```python
from build123d import *

# Parameters (mm, degrees)
F1_DEPTH = 6.35
F4_DEPTH = 6.35


with BuildPart() as f1:
    # F0 (on Top) → F1 (new body)
    with BuildSketch(Plane.XY):
        Polygon((12.7, -7.3323484187), (12.7, 7.3323484187), (0, 14.6646968374), (-12.7, 7.3323484187), (-12.7, -7.3323484187), (0, -14.6646968374), align=None)
    extrude(amount=F1_DEPTH)

    # F3 (on face) → F4 (join, through all)
    with BuildSketch(Plane(origin=(0, 0, 0), x_dir=(1, 0, 0), z_dir=(0, 0, -1))):
        with BuildLine():
            ThreePointArc((4.3930360984, 12.1283762634), (6.2703188288, 14.5276326774), (6.9390436724, 17.4997411668))
            ThreePointArc((6.9390436724, 17.4997411668), (-2.9721084894, 23.7700599956), (-4.3930360984, 12.1283762634))
            Line((-4.3930360984, 12.1283762634), (-1.9827005664, 13.5199841317))
            ThreePointArc((-1.9827005664, 13.5199841317), (-2.3402873387, 21.2802996927), (4.4462981901, 17.4997411668))
            ThreePointArc((4.4462981901, 17.4997411668), (3.7805585258, 15.1594538282), (1.9827005664, 13.5199841317))
            Line((1.9827005664, 13.5199841317), (4.3930360984, 12.1283762634))
        make_face()
    extrude(amount=-F4_DEPTH)


solid = f1.part
```
Source: CAD feature listing. Evaluate the final solid. Frame: model axes, mm. A direction names the side the tool comes from. Round coordinates to 2 decimals unless told otherwise and drop trailing zeros. Write each loop counter-clockwise with the first axis right and the second up, starting at its lowest first coordinate (ties: lowest second). Pieces come first, ordered by that corner, then holes. Notation, with made-up numbers: M -20,31.5 L -16,31.5 A31 cw -16,60.5 Z; hole C 23,53.25 d6. An arc over 180 degrees is marked long. Answer as a JSON object with one key per item and string values. Group by question number.
(1) Section query A-A on z = 5.5. Output: boundary loops of the cut face in (x, y), then the cut area to 3 significant figures.
(2) Section query D-D on x = 8.75. Output: boundary loops of the cut face in (y, z), then the cut area to 3 significant figures.
(3) Mould query, pull axis X, two halves, no side actions, for faces 4 (the flat face through (0.98, -14.1, 3.13)), 5 (the flat face through (0, 0, 0)), 6 (the flat face through (-1.01, -14.08, 3.13)), 7 (the flat face through (12.7, 0, 3)). Classes: +X half, -X half, draft (parallel to the pull), parting line (faces both ways), or undercut.
(4) First-contact query: pin 1 (1.5 mm diameter, centred on x = 3.5, z = 3.5, fed in from -Y); pin 2 (1 mm diameter, centred on x = 1.5, z = 0.5, fed in from +Y). Flat tips, straight axial feed; report the tip coordinate or a pass-through.
(5) Section query B-B on x = 0.5. Output: boundary loops of the cut face in (y, z).
(6) Section query C-C on x = -9.25. Output: boundary loops of the cut face in (y, z), then the cut area to 3 significant figures.
(7) Ray query, line 1 (Y direction, x = 0, z = 2.75); line 2 (X direction, y = -20, z = 4); line 3 (Y direction, x = 2.25, z = 1.25). Return the intervals inside material, ascending. Write a range as [from, to].
(8) Reachability of faces 1 (the flat face through (-8.6, -9.7, 3.1)), 2 (the flat face through (-6.26, 11.05, 3.13)), 3 (the flat face through (8.488, -9.764, 3.131)) from +Z, -Z, +X, -X, +Y, -Y: full face, straight path, thin tool, end or side. Return the list, or none.
Computed values:
{
 "1": {"outline": "M -12.7,-7.33 L -4.39,-12.13 A6.94 ccw long 4.39,-12.13 L 12.7,-7.33 L 12.7,7.33 L 0,14.66 L -12.7,7.33 Z; hole M -1.98,-13.52 A4.45 ccw long 1.98,-13.52 L 0,-14.66 Z", "area": "631 mm^2"},
 "2": {"outline": "M -9.61,0 L 9.61,0 L 9.61,6.35 L -9.61,6.35 Z", "area": "122 mm^2"},
 "3": {"face 4": "undercut", "face 5": "draft", "face 6": "undercut", "face 7": "+X half"},
 "4": {"pin 1": "y = -23.87", "pin 2": "y = 14.09"},
 "5": {"outline": "M -24.42,0 L -21.92,0 L -21.92,6.35 L -24.42,6.35 Z; M -14.38,0 L 14.38,0 L 14.38,6.35 L -14.38,6.35 Z"},
 "6": {"outline": "M -9.32,0 L 9.32,0 L 9.32,6.35 L -9.32,6.35 Z", "area": "118 mm^2"},
 "7": {"line 1": "[-24.44, -21.95], [-14.66, 14.66]", "line 2": "[-6.47, -3.68], [3.68, 6.47]", "line 3": "[-24.06, -21.33], [-13.66, 13.37]"},
 "8": {"face 1": "+Z, -Z, -X", "face 2": "+Z, -Z, -X, +Y", "face 3": "+Z, -Z, +X"}
}
